The model under review builds one solid part; all positions refer to its coordinate system, in mm. A direction names the side the tool comes from. Coordinates: 2 decimals unless noted, no trailing zeros. Order: outer loops, then holes, each group sorted by start corner. A loop starts at its lowest first (then second) coordinate and runs counter-clockwise, first axis right, second up.
from build123d import *

# Parameters (mm, degrees)
SKETCH1_R           = 1.5
BOSS_EXTRUDE1_DEPTH = 4
SKETCH2_R           = 1.5
CUT_EXTRUDE1_DEPTH  = 4
SKETCH8_R           = 1.5
CUT_EXTRUDE5_DEPTH  = 85.436165497
SKETCH9_R           = 1.5
CUT_EXTRUDE6_DEPTH  = 10
CUT_EXTRUDE7_DEPTH  = 10


with BuildPart() as part:
    # Sketch1 → Boss-Extrude1 (new body)
    with BuildSketch(Plane(origin=(0, 0, 0), x_dir=(1, 0, 0), z_dir=(0, 1, 0))):
        with BuildLine():
            Line((-48.31716421, 29.901561441), (-41.781630304, 36.437095347))
            ThreePointArc((-41.781630304, 36.437095347), (-40.15951356, 37.520959103), (-38.246096398, 37.901561441))
            Line((-38.246096398, 37.901561441), (37.753903602, 37.901561441))
            ThreePointArc((37.753903602, 37.901561441), (39.667320764, 37.520959103), (41.289437508, 36.437095347))
            Line((41.289437508, 36.437095347), (47.824971414, 29.901561441))
            Line((47.824971414, 29.901561441), (66.753903602, 29.901561441))
            ThreePointArc((66.753903602, 29.901561441), (72.410757852, 27.55841569), (74.753903602, 21.901561441))
            Line((74.753903602, 21.901561441), (74.753903602, -22.098438559))
            ThreePointArc((74.753903602, -22.098438559), (72.410757852, -27.755292809), (66.753903602, -30.098438559))
            Line((66.753903602, -30.098438559), (47.824971414, -30.098438559))
            Line((47.824971414, -30.098438559), (41.289437508, -36.633972465))
            ThreePointArc((41.289437508, -36.633972465), (39.667320764, -37.717836222), (37.753903602, -38.098438559))
            Line((37.753903602, -38.098438559), (-38.246096398, -38.098438559))
            ThreePointArc((-38.246096398, -38.098438559), (-40.15951356, -37.717836222), (-41.781630304, -36.633972465))
            Line((-41.781630304, -36.633972465), (-48.31716421, -30.098438559))
            Line((-48.31716421, -30.098438559), (-67.246096398, -30.098438559))
            ThreePointArc((-67.246096398, -30.098438559), (-72.902950647, -27.755292809), (-75.246096398, -22.098438559))
            Line((-75.246096398, -22.098438559), (-75.246096398, 21.901561441))
            ThreePointArc((-75.246096398, 21.901561441), (-72.902950647, 27.55841569), (-67.246096398, 29.901561441))
            Line((-67.246096398, 29.901561441), (-48.31716421, 29.901561441))
        make_face()
        with Locations(Location((-7.246096398, 22, 0), (0, 0, 270))):
            Circle(SKETCH1_R, mode=Mode.SUBTRACT)
        with Locations(Location((54.753903602, 22, 0), (0, 0, 90))):
            Circle(SKETCH1_R, mode=Mode.SUBTRACT)
        with Locations(Location((54.753903602, -22, 0), (0, 0, 270))):
            Circle(SKETCH1_R, mode=Mode.SUBTRACT)
        with Locations(Location((-7.246096398, -22, 0), (0, 0, 90))):
            Circle(SKETCH1_R, mode=Mode.SUBTRACT)
    extrude(amount=-BOSS_EXTRUDE1_DEPTH)

    # Sketch2 → Cut-Extrude1 (cut)
    with BuildSketch(Plane(origin=(0, 0, 0), x_dir=(1, 0, 0), z_dir=(0, 1, 0))):
        with Locations(Location((-42.5, 15.539099556, 0), (0, 0, 270))):
            Circle(SKETCH2_R)
        with Locations(Location((-66, 15.539099556, 0), (0, 0, 270))):
            Circle(SKETCH2_R)
        with Locations(Location((-66, -14.460900444, 0), (0, 0, 270))):
            Circle(SKETCH2_R)
        with Locations(Location((-42.5, -14.460900444, 0), (0, 0, 270))):
            Circle(SKETCH2_R)
        with Locations(Location((66, 15.539099556, 0), (0, 0, 90))):
            Circle(SKETCH2_R)
        with Locations(Location((66, -14.460900444, 0), (0, 0, 90))):
            Circle(SKETCH2_R)
        with Locations(Location((42.5, -14.460900444, 0), (0, 0, 90))):
            Circle(SKETCH2_R)
        with Locations(Location((42.5, 15.539099556, 0), (0, 0, 90))):
            Circle(SKETCH2_R)
    extrude(amount=-CUT_EXTRUDE1_DEPTH, mode=Mode.SUBTRACT)

    # Sketch8 → Cut-Extrude5 (cut, through all)
    with BuildSketch(Plane.XZ.offset(4)):
        with Locations(Location((-40.31716421, -29.901561441, 0), (0, 0, 270))):
            Circle(SKETCH8_R)
        with Locations(Location((39.824971414, -29.901561441, 0), (0, 0, 90))):
            Circle(SKETCH8_R)
        with Locations(Location((39.824971414, 30.098438559, 0), (0, 0, 270))):
            Circle(SKETCH8_R)
        with Locations(Location((-40.31716421, 30.098438559, 0), (0, 0, 90))):
            Circle(SKETCH8_R)
    extrude(amount=-CUT_EXTRUDE5_DEPTH, mode=Mode.SUBTRACT)

    # Sketch9 → Cut-Extrude6 (cut)
    with BuildSketch(Plane(origin=(0, 0, 0), x_dir=(1, 0, 0), z_dir=(0, 1, 0))):
        with Locations(Location((-34.747808705, -15, 0), (0, 0, 270))):
            Circle(SKETCH9_R)
        with Locations(Location((-18.747808705, 15, 0), (0, 0, 270))):
            Circle(SKETCH9_R)
    extrude(amount=-CUT_EXTRUDE6_DEPTH, mode=Mode.SUBTRACT)

    # Sketch10 → Cut-Extrude7 (cut)
    with BuildSketch(Plane(origin=(0, 0, 0), x_dir=(1, 0, 0), z_dir=(0, 1, 0))):
        with BuildLine():
            Line((15.753903602, 22), (31.753903602, 22))
            ThreePointArc((31.753903602, 22), (32.461010383, 22.292893219), (32.753903602, 23))
            Line((32.753903602, 23), (32.753903602, 26))
            ThreePointArc((32.753903602, 26), (32.461010383, 26.707106781), (31.753903602, 27))
            Line((31.753903602, 27), (15.753903602, 27))
            ThreePointArc((15.753903602, 27), (15.046796821, 26.707106781), (14.753903602, 26))
            Line((14.753903602, 26), (14.753903602, 23))
            ThreePointArc((14.753903602, 23), (15.046796821, 22.292893219), (15.753903602, 22))
        make_face()
        with BuildLine():
            Line((-32.256634528, -26.962874327), (-16.256690018, -27.005012975))
            ThreePointArc((-16.256690018, -27.005012975), (-15.548814306, -26.713983054), (-15.25405982, -26.007650108))
            Line((-15.25405982, -26.007650108), (-15.246158824, -23.007660513))
            ThreePointArc((-15.246158824, -23.007660513), (-15.537188744, -22.299784801), (-16.24352169, -22.005030315))
            Line((-16.24352169, -22.005030315), (-32.243466201, -21.962891667))
            ThreePointArc((-32.243466201, -21.962891667), (-32.951341912, -22.253921588), (-33.246096398, -22.960254534))
            Line((-33.246096398, -22.960254534), (-33.253997394, -25.960244129))
            ThreePointArc((-33.253997394, -25.960244129), (-32.962967474, -26.668119841), (-32.256634528, -26.962874327))
        make_face()
        with BuildLine():
            Line((32.753903602, -22.960254534), (32.761804599, -25.960244129))
            ThreePointArc((32.761804599, -25.960244129), (32.470774678, -26.668119841), (31.764441732, -26.962874327))
            Line((31.764441732, -26.962874327), (15.764497222, -27.005012975))
            ThreePointArc((15.764497222, -27.005012975), (15.05662151, -26.713983054), (14.761867024, -26.007650108))
            Line((14.761867024, -26.007650108), (14.753966028, -23.007660513))
            ThreePointArc((14.753966028, -23.007660513), (15.044995948, -22.299784801), (15.751328894, -22.005030315))
            Line((15.751328894, -22.005030315), (31.751273405, -21.962891667))
            ThreePointArc((31.751273405, -21.962891667), (32.459149116, -22.253921588), (32.753903602, -22.960254534))
        make_face()
        with BuildLine():
            Line((-16.246096398, 27), (-32.246096398, 27))
            ThreePointArc((-32.246096398, 27), (-32.953203179, 26.707106781), (-33.246096398, 26))
            Line((-33.246096398, 26), (-33.246096398, 23))
            ThreePointArc((-33.246096398, 23), (-32.953203179, 22.292893219), (-32.246096398, 22))
            Line((-32.246096398, 22), (-16.246096398, 22))
            ThreePointArc((-16.246096398, 22), (-15.538989617, 22.292893219), (-15.246096398, 23))
            Line((-15.246096398, 23), (-15.246096398, 26))
            ThreePointArc((-15.246096398, 26), (-15.538989617, 26.707106781), (-16.246096398, 27))
        make_face()
    extrude(amount=-CUT_EXTRUDE7_DEPTH, mode=Mode.SUBTRACT)


solid = part.part
(1) The part is to be moulded in two halves that separate along Z. For faces 5 (the face through (-58, -2, -29.902)), 6 (the face through (64.74, -1.97, -16.35)), 7 (the face through (1, 0, 0)), say which applies: +Z half, -Z half, draft (parallel to the pull), parting line (faces both ways), or undercut.
(2) Consider section A-A (x = -25.5). Give the boundary of the cut face in (y, z).
(3) Tool access review of faces 1 (the face through (-24, -2, -22)), 2 (the face through (57, -2, 30.098)), 3 (the face through (-58, -2, 30.098)), 4 (the face through (-75.246, -2, 0)): name each direction out of +Z, -Z, +X, -X, +Y, -Y from which nothing blocks a thin tool from reaching the whole face with its end or side.
(4) Insertion check: pin 1 Ø1.2 at (x, y) = (56, -2.5) entering from -Z; pin 2 Ø3.5 at (x, z) = (66, -15.54) entering from -Y; pin 3 Ø2 at (x, y) = (-61.5, -1.5) entering from +Z. Each pin has a flat end and moves straight along its axis. Give the tip position at first contact, or say it passes through.
(5) Consider section B-B (y = -2.15). Give the number of separate pieces and of enclosed holes in the cut face, then the cut area to 3 significant figures.
(6) Wall thickness on line 1 (Z direction, x = -16, y = -2.05); line 2 (X direction, y = -0.7, z = -23); line 3 (X direction, y = -3.15, z = -30): over which ranges is each line inside the solid? List them lowest first.
Findings:
1. face 5: -Z half
1. face 6: undercut
1. face 7: draft
2. outline: (-4, -37.9) - (0, -37.9) - (0, -27) - (-4, -27) - close; (-4, -22) - (0, -22) - (0, 21.98) - (-4, 21.98) - close; (-4, 26.98) - (0, 26.98) - (0, 38.1) - (-4, 38.1) - close
3. face 1: +Y, -Y
3. face 2: +Z, +X, +Y, -Y
3. face 3: +Z, -X, +Y, -Y
3. face 4: +Z, -Z, -X, +Y, -Y
4. pin 1: stops at z = -29.9
4. pin 2: stops at y = -4
4. pin 3: stops at z = 30.1
5. separate pieces: 1
5. enclosed holes: 22
5. area: 9,870 mm2
6. line 1: z = -37.9 to -26.97, -22.03 to 22.04, 26.97 to 38.1
6. line 2: x = -75.17 to -33.25, -15.25 to -8.36, -6.13 to 14.75, 32.75 to 53.64, 55.87 to 74.68
6. line 3: x = -48.22 to -41.81, -38.82 to 38.33, 41.32 to 47.73
